CAD build for the part. Positions are in the model's coordinates, mm. A direction names the side the tool comes from. Round coordinates to 2 decimals unless told otherwise and drop trailing zeros. Loops run counter-clockwise (first coordinate to the right, second up) from the corner with the lowest first, then second, coordinate; pieces in that order, holes last.
Autodesk Inventor part; units mm, degrees
ref_plane "YZ Plane" through (0, 0, 0) normal (1, 0, 0) x (0, 1, 0)
ref_plane "XZ Plane" through (0, 0, 0) normal (0, 1, 0) x (-1, 0, 0)
ref_plane "XY Plane" through (0, 0, 0) normal (0, 0, 1) x (1, 0, 0)
sketch "Skizze1" plane through (0, 0, 0) normal (0, 0, 1) x (1, 0, 0)
  line L0 (-41.5, 35.6804) -> (-41.5, -22.9) construction
  line L1 (-41.5, -22.9) -> (-43.9777, -22.9) construction
  line L2 (-43.9777, -22.9) -> (-43.9777, 35.6804) construction
  line L3 (-43.9777, 35.6804) -> (-41.5, 35.6804) construction
  line L4 (-47.5, 35.6804) -> (-47.5, -0.041) construction
  line L5 (-47.5, -0.041) -> (-49.9777, -0.041) construction
  line L6 (-49.9777, -0.041) -> (-49.9777, 35.6804) construction
  line L7 (-49.9777, 35.6804) -> (-47.5, 35.6804) construction
  circle A0 centre (-47.5, -3) radius 1.35 construction
  line L8 (36.5, 27.1) -> (36.5, -35.7623) construction
  line L9 (36.5, -35.7623) -> (34.0223, -35.7623) construction
  line L10 (34.0223, -35.7623) -> (34.0223, 27.1) construction
  line L11 (34.0223, 27.1) -> (36.5, 27.1) construction
  line L12 (30.5, -25.9706) -> (30.5, -35.7623) construction
  line L13 (30.5, -35.7623) -> (28.0223, -35.7623) construction
  line L14 (28.0223, -35.7623) -> (28.0223, -25.9706) construction
  line L15 (28.0223, -25.9706) -> (30.5, -25.9706) construction
  line L16 (18.5, -28.5) -> (18.5, -35.7623) construction
  line L17 (18.5, -35.7623) -> (16.0223, -35.7623) construction
  line L18 (16.0223, -35.7623) -> (16.0223, -28.5) construction
  line L19 (16.0223, -28.5) -> (18.5, -28.5) construction
  line L20 (-29.5, -16.7561) -> (-29.5, -22.9) construction
  line L21 (-29.5, -22.9) -> (-31.9777, -22.9) construction
  line L22 (-31.9777, -22.9) -> (-31.9777, -16.7561) construction
  line L23 (-31.9777, -16.7561) -> (-29.5, -16.7561) construction
  line L24 (-25.9777, 30.1243) -> (-25.9777, 35.6804) construction
  line L25 (-25.9777, 35.6804) -> (-23.5, 35.6804) construction
  line L26 (-23.5, 35.6804) -> (-23.5, 30.1243) construction
  line L27 (-23.5, 30.1243) -> (-25.9777, 30.1243) construction
  line L28 (16.0223, 31.6466) -> (16.0223, 35.6804) construction
  line L29 (16.0223, 35.6804) -> (18.5, 35.6804) construction
  line L30 (18.5, 35.6804) -> (18.5, 31.6466) construction
  line L31 (18.5, 31.6466) -> (16.0223, 31.6466) construction
  line L32 (-5.5, -32.1312) -> (-5.5, -35.7623) construction
  line L33 (-5.5, -35.7623) -> (-7.9777, -35.7623) construction
  line L34 (-7.9777, -35.7623) -> (-7.9777, -32.1312) construction
  line L35 (-7.9777, -32.1312) -> (-5.5, -32.1312) construction
  line L36 (10.0223, 32.8979) -> (10.0223, 35.6804) construction
  line L37 (10.0223, 35.6804) -> (12.5, 35.6804) construction
  line L38 (12.5, 35.6804) -> (12.5, 32.8979) construction
  line L39 (12.5, 32.8979) -> (10.0223, 32.8979) construction
  line L40 (-7.9777, 33.0955) -> (-7.9777, 35.6804) construction
  line L41 (-7.9777, 35.6804) -> (-5.5, 35.6804) construction
  line L42 (-5.5, 35.6804) -> (-5.5, 33.0955) construction
  line L43 (-5.5, 33.0955) -> (-7.9777, 33.0955) construction
  line L44 (0.5, -33.9467) -> (0.5, -35.7623) construction
  line L45 (0.5, -35.7623) -> (-1.9777, -35.7623) construction
  line L46 (-1.9777, -35.7623) -> (-1.9777, -33.9467) construction
  line L47 (-1.9777, -33.9467) -> (0.5, -33.9467) construction
  line L48 (-1.9777, 34.0902) -> (-1.9777, 35.6804) construction
  line L49 (-1.9777, 35.6804) -> (0.5, 35.6804) construction
  line L50 (0.5, 35.6804) -> (0.5, 34.0902) construction
  line L51 (0.5, 34.0902) -> (-1.9777, 34.0902) construction
  line L52 (6.5, -33.9467) -> (6.5, -35.7623) construction
  line L53 (6.5, -35.7623) -> (4.0223, -35.7623) construction
  line L54 (4.0223, -35.7623) -> (4.0223, -33.9467) construction
  line L55 (4.0223, -33.9467) -> (6.5, -33.9467) construction
  line L56 (4.0223, 32.8979) -> (4.0223, 35.6804) construction
  line L57 (4.0223, 35.6804) -> (6.5, 35.6804) construction
  line L58 (6.5, 35.6804) -> (6.5, 32.8979) construction
  line L59 (6.5, 32.8979) -> (4.0223, 32.8979) construction
  line L60 (-13.9777, 32.5) -> (-13.9777, 35.6804) construction
  line L61 (-13.9777, 35.6804) -> (-11.5, 35.6804) construction
  line L62 (-11.5, 35.6804) -> (-11.5, 32.5) construction
  line L63 (-11.5, 32.5) -> (-13.9777, 32.5) construction
  line L64 (12.5, -32.1312) -> (12.5, -35.7623) construction
  line L65 (12.5, -35.7623) -> (10.0223, -35.7623) construction
  line L66 (10.0223, -35.7623) -> (10.0223, -32.1312) construction
  line L67 (10.0223, -32.1312) -> (12.5, -32.1312) construction
  line L68 (-19.9777, 31.3064) -> (-19.9777, 35.6804) construction
  line L69 (-19.9777, 35.6804) -> (-17.5, 35.6804) construction
  line L70 (-17.5, 35.6804) -> (-17.5, 31.3064) construction
  line L71 (-17.5, 31.3064) -> (-19.9777, 31.3064) construction
  line L72 (22.0223, 30) -> (22.0223, 35.6804) construction
  line L73 (22.0223, 35.6804) -> (24.5, 35.6804) construction
  line L74 (24.5, 35.6804) -> (24.5, 30) construction
  line L75 (24.5, 30) -> (22.0223, 30) construction
  line L76 (-29.5, 27.1) -> (-29.5, 20.9081) construction
  line L77 (-29.5, 20.9081) -> (-31.9777, 20.9081) construction
  line L78 (-31.9777, 20.9081) -> (-31.9777, 27.1) construction
  line L79 (-31.9777, 27.1) -> (-29.5, 27.1) construction
  line L80 (24.5, -28.5) -> (24.5, -35.7623) construction
  line L81 (24.5, -35.7623) -> (22.0223, -35.7623) construction
  line L82 (22.0223, -35.7623) -> (22.0223, -28.5) construction
  line L83 (22.0223, -28.5) -> (24.5, -28.5) construction
  line L84 (-49.9777, -22.9) -> (-49.9777, -6.1402) construction
  line L85 (-49.9777, -6.1402) -> (-47.5, -6.1402) construction
  line L86 (-47.5, -6.1402) -> (-47.5, -22.9) construction
  line L87 (-47.5, -22.9) -> (-49.9777, -22.9) construction
  line L88 (46.0223, -27.1) -> (46.0223, 35.6804) construction
  line L89 (46.0223, 35.6804) -> (48.5, 35.6804) construction
  line L90 (48.5, 35.6804) -> (48.5, -27.1) construction
  line L91 (48.5, -27.1) -> (46.0223, -27.1) construction
  line L92 (40.0223, 35.6804) -> (42.5, 35.6804) construction
  line L93 (42.5, 35.6804) -> (42.5, -35.7623) construction
  line L94 (42.5, -35.7623) -> (40.0223, -35.7623) construction
  line L95 (40.0223, -35.7623) -> (40.0223, 35.6804) construction
  circle A1 centre (25, 25) radius 2.1 construction
  circle A2 centre (-25, 25) radius 2.1 construction
  circle A3 centre (-25, -25) radius 2.1 construction
  circle A4 centre (25, -25) radius 2.1 construction
  circle A5 centre (32, 32.5) radius 1.35 construction
  circle A6 centre (-30, 32.5) radius 1.35 construction
  circle A7 centre (47.5, -32.5) radius 1.35 construction
  line L96 (-35.5, 35.6804) -> (-35.5, -22.9) construction
  line L97 (-35.5, -22.9) -> (-37.9777, -22.9) construction
  line L98 (-37.9777, -22.9) -> (-37.9777, 35.6804) construction
  line L99 (-37.9777, 35.6804) -> (-35.5, 35.6804) construction
  line L100 (-52.5, -24.5) -> (-52.5, 37.5) construction
  line L101 (-52.5, -24.5) -> (-32.8176, -24.5) construction
  arc A8 (-32.8176, -24.5) -> (-11.4624, -29.9989) centre (-10.5668, 17.6958) ccw construction
  arc A9 (-9.5, -31.9985) -> (-11.4624, -29.9989) centre (-11.5, -31.9985) ccw construction
  line L102 (-9.5, -31.9985) -> (-9.5, -37.5) construction
  line L103 (52.5, -37.5) -> (-9.5, -37.5) construction
  line L104 (52.5, 37.5) -> (52.5, -37.5) construction
  line L105 (-52.5, 37.5) -> (52.5, 37.5) construction
  circle A10 centre (0, 0) radius 32 construction
  line L106 (-32, 32) -> (32, 32)
  line L107 (32, 32) -> (32, -32)
  line L108 (32, -32) -> (-32, -32)
  line L109 (-32, -32) -> (-32, 32)
  line L110 (-32, 32) -> (32, -32) construction
  line L111 (32, 32) -> (-32, -32) construction
extrude "Extrusion1" add sketch "Skizze1" along normal blind 3
sketch "Skizze2" plane through (0, 0, 3) normal (0, 0, 1) x (1, 0, 0)
  circle A0 centre (0, 0) radius 30
  circle A1 centre (25, 25) radius 2.1
  circle A2 centre (-25, 25) radius 2.1
  circle A3 centre (-25, -25) radius 2.1
  circle A4 centre (25, -25) radius 2.1
extrude "Extrusion2" cut sketch "Skizze2" against normal through all
sketch "Skizze3" plane through (0, 0, 3) normal (0, 0, 1) x (1, 0, 0)
  line L0 (28.0978, 30) -> (26.0978, 30)
  line L1 (26.0978, 30) -> (26.0978, -29.358)
  line L2 (26.0978, -29.358) -> (28.0978, -29.358)
  line L3 (28.0978, -29.358) -> (28.0978, 30)
  line L4 (32, 32) -> (-32, 32) construction
  line L5 (23.0978, 30) -> (21.0978, 30)
  line L6 (21.0978, 30) -> (21.0978, -29.358)
  line L7 (21.0978, -29.358) -> (23.0978, -29.358)
  line L8 (23.0978, -29.358) -> (23.0978, 30)
  line L9 (18.0978, 30) -> (16.0978, 30)
  line L10 (16.0978, 30) -> (16.0978, -29.358)
  line L11 (16.0978, -29.358) -> (18.0978, -29.358)
  line L12 (18.0978, -29.358) -> (18.0978, 30)
  line L13 (13.0978, 30) -> (11.0978, 30)
  line L14 (11.0978, 30) -> (11.0978, -29.358)
  line L15 (11.0978, -29.358) -> (13.0978, -29.358)
  line L16 (13.0978, -29.358) -> (13.0978, 30)
  line L17 (8.0978, 30) -> (6.0978, 30)
  line L18 (6.0978, 30) -> (6.0978, -29.358)
  line L19 (6.0978, -29.358) -> (8.0978, -29.358)
  line L20 (8.0978, -29.358) -> (8.0978, 30)
  line L21 (3.0978, 30) -> (1.0978, 30)
  line L22 (1.0978, 30) -> (1.0978, -29.358)
  line L23 (1.0978, -29.358) -> (3.0978, -29.358)
  line L24 (3.0978, -29.358) -> (3.0978, 30)
  line L25 (-1.9022, 30) -> (-3.9022, 30)
  line L26 (-3.9022, 30) -> (-3.9022, -29.358)
  line L27 (-3.9022, -29.358) -> (-1.9022, -29.358)
  line L28 (-1.9022, -29.358) -> (-1.9022, 30)
  line L29 (-6.9022, 30) -> (-8.9022, 30)
  line L30 (-8.9022, 30) -> (-8.9022, -29.358)
  line L31 (-8.9022, -29.358) -> (-6.9022, -29.358)
  line L32 (-6.9022, -29.358) -> (-6.9022, 30)
  line L33 (-11.9022, 30) -> (-13.9022, 30)
  line L34 (-13.9022, 30) -> (-13.9022, -29.358)
  line L35 (-13.9022, -29.358) -> (-11.9022, -29.358)
  line L36 (-11.9022, -29.358) -> (-11.9022, 30)
  line L37 (-16.9022, 30) -> (-18.9022, 30)
  line L38 (-18.9022, 30) -> (-18.9022, -29.358)
  line L39 (-18.9022, -29.358) -> (-16.9022, -29.358)
  line L40 (-16.9022, -29.358) -> (-16.9022, 30)
  line L41 (-21.9022, 30) -> (-23.9022, 30)
  line L42 (-23.9022, 30) -> (-23.9022, -29.358)
  line L43 (-23.9022, -29.358) -> (-21.9022, -29.358)
  line L44 (-21.9022, -29.358) -> (-21.9022, 30)
  line L45 (-26.9022, 30) -> (-28.9022, 30)
  line L46 (-28.9022, 30) -> (-28.9022, -29.358)
  line L47 (-28.9022, -29.358) -> (-26.9022, -29.358)
  line L48 (-26.9022, -29.358) -> (-26.9022, 30)
  point P0 (0, 0)
  dimension "d4" = 2
  dimension "d7" = 5
extrude "Extrusion3" add sketch "Skizze3" against normal blind 3
sketch "Skizze4" plane through (0, 0, 3) normal (0, 0, 1) x (1, 0, 0)
  arc A0 (-23.9022, 26.7902) -> (-26.9022, 25.8897) centre (-25, 25) ccw
  arc A1 (26.0978, 26.7902) -> (23.0978, 25.8897) centre (25, 25) ccw
  arc A2 (26.0978, -23.2098) -> (23.0978, -24.1103) centre (25, -25) ccw
  arc A3 (-23.9022, -23.2098) -> (-26.9022, -24.1103) centre (-25, -25) ccw
  circle A4 centre (-25, 25) radius 2.1
  circle A5 centre (25, 25) radius 2.1
  circle A6 centre (25, -25) radius 2.1
  circle A7 centre (-25, -25) radius 2.1
  point P0 (0, 0)
extrude "Extrusion4" cut sketch "Skizze4" against normal blind 3
fillet "Rundung1" radius 10 4 edges at (32, 32, 1.5) (32, -32, 1.5) (-32, 32, 1.5) (-32, -32, 1.5)
properties part number "Fan_blend"
Item 1: Cut at D-D (z = 1.4). State how many separate pieces and enclosed holes the cut face has, plus the area to 3 significant figures.
Verdict:
separate pieces: 1
enclosed holes: 15
area: 2,260 mm2
Item 2: Cut at A-A (x = -25). List the corners of the cut face in (y, z).
Verdict:
outline: (-31.54, 0) - (-27.1, 0) - (-27.1, 3) - (-31.54, 3) - close; (-22.9, 0) - (-16.58, 0) - (-16.58, 3) - (-22.9, 3) - close; (16.58, 0) - (22.9, 0) - (22.9, 3) - (16.58, 3) - close; (27.1, 0) - (31.54, 0) - (31.54, 3) - (27.1, 3) - close
Item 3: 3-axis set-ups, long thin cutter, end or side, ignore diameter. For faces 1 (the flat face through (26.098, 0, 2)), 2 (the cylindrical face through (29.15, 28.99, 1.52)): which of +Z, -Z, +X, -X, +Y, -Y reach the whole face in a straight line?
Verdict:
face 1: +Z, -Z
face 2: +Z, -Z, +X, +Y
Item 4: Mould opens along X. For faces 3 (the cylindrical face through (-29.15, -28.99, 1.52)), 4 (the cylindrical face through (14.643, 26.184, 1.521)), 5 (the flat face through (32, 0, 1)) say: released by +X, released by -X, zero draft, split by the parting line, or undercut.
Verdict:
face 3: released by -X
face 4: undercut
face 5: released by +X
Item 5: Cut at B-B (x = -11). List the corners of the cut face in (y, z).
Verdict:
outline: (-32, 0) - (-27.91, 0) - (-27.91, 3) - (-32, 3) - close; (27.91, 0) - (32, 0) - (32, 3) - (27.91, 3) - close
Item 6: Wall check: L1, parallel to Y at x = -24, z = 1.85; L2, parallel to Y at x = -25, z = 1.7; L3, parallel to X at y = -27.5, z = 1.2. Give the ranges that are in metal, low to high.
Verdict:
L1: y = -31.8 to -26.85, -23.15 to -18, 18 to 23.15, 26.85 to 31.8
L2: y = -31.54 to -27.1, -22.9 to -16.58, 16.58 to 22.9, 27.1 to 31.54
L3: x = -30.35 to -11.9, -8.9 to -6.9, -3.9 to -1.9, 1.1 to 3.1, 6.1 to 8.1, 11.1 to 30.35
Item 7: Flat gauge pin, fed straight in: P1, Ø3, axis at x = 5, y = -17, coming from the -Z side. Where does the tip first touch, or does it go through?
Verdict:
P1: stops at z = 0
Item 8: Cut at C-C (x = 24.5). List the corners of the cut face in (y, z).
Verdict:
outline: (-31.68, 0) - (-27.04, 0) - (-27.04, 3) - (-31.68, 3) - close; (-22.96, 0) - (-17.31, 0) - (-17.31, 3) - (-22.96, 3) - close; (17.31, 0) - (22.96, 0) - (22.96, 3) - (17.31, 3) - close; (27.04, 0) - (31.68, 0) - (31.68, 3) - (27.04, 3) - close
